Here's the drawing with two shaded views (mm, measured from the low corner). I have some questions. A direction names the side the tool comes from. Give positions to 0.01 mm unless a question says otherwise; leave off trailing zeros. Order: outer loops, then holes, each group sorted by start corner. A loop starts at its lowest first (then second) coordinate and runs counter-clockwise, first axis right, second up. Notation, with made-up numbers: (3.25, 45.25) - (53.25, 45.25) arc R17 cw to (53.25, 62.25) - close; hole circle Ø7 at (-36, 37). An arc over 180 degrees is marked (long way). Use one line per item in the form item = value. Start each with the question number.
1) Please list where these lines run through material, in increasing order: probe 1 along Y at (x, z) = (30, 11.5); probe 2 along Y at (x, z) = (30, 6.5); probe 3 along Z at (x, y) = (50, 8).
2) Which directions (+Z, -Z, +X, -X, +Y, -Y) give clear straight access to the entire face, cutting with the end or side of a thin tool? Please do the marked faces 1, 2 and 3.
3) Suppose I cut it at A-A, the plane y = 30. Write out the boundary of the cut face in (x, z).
4) Suppose I cut it at C-C, the plane z = 11.5. Write out the boundary of the cut face in (x, y), and give its area (3 significant figures).
5) Suppose I cut it at B-B, the plane z = 23.5. Write out the boundary of the cut face in (x, y).
6) We'd pull the mould along X, two halves only. Please class the marked faces 4, 5 and 6: released by +X, released by -X, zero draft, split by the parting line, or undercut.
7) For pin 1 (12 mm diameter, centred on x = 10, z = 13, fed in from +Y); pin 2 (1.5 mm diameter, centred on x = 32.5, z = 15, fed in from +Y); pin 3 (8 mm diameter, centred on x = 41, y = 37, fed in from +Z), each with a flat end and sliding along its axis, tell me the tip position at first contact or that it passes through.
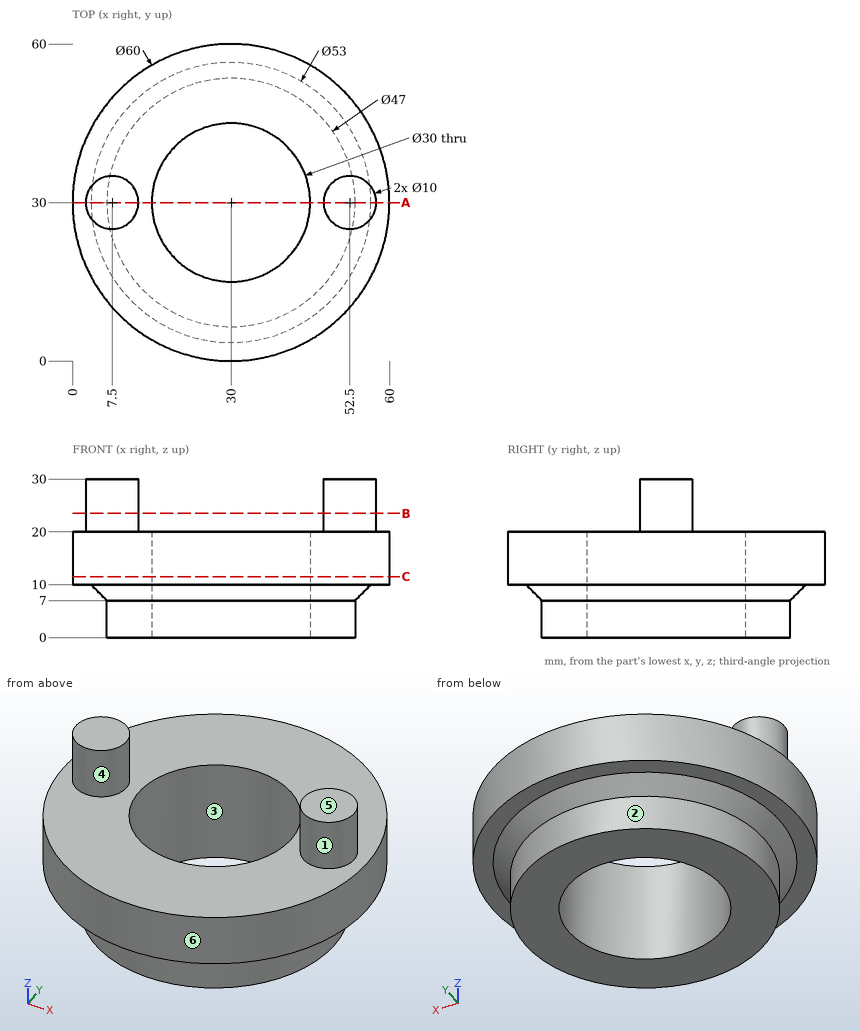
Result sheet:
q1.probe_1 = 0 to 15, 45 to 60
q1.probe_2 = 6.5 to 15, 45 to 53.5
q1.probe_3 = 10 to 20
q2.face_1 = +Z
q2.face_2 = -Z
q2.face_3 = +Z, -Z
q3.outline = (0, 10) - (3.5, 10) - (6.5, 7) - (6.5, 0) - (15, 0) - (15, 20) - (12.5, 20) - (12.5, 30) - (2.5, 30) - (2.5, 20) - (0, 20) - close; (45, 0) - (53.5, 0) - (53.5, 7) - (56.5, 10) - (60, 10) - (60, 20) - (57.5, 20) - (57.5, 30) - (47.5, 30) - (47.5, 20) - (45, 20) - close
q4.outline = circle Ø60 at (30, 30); hole circle Ø30 at (30, 30)
q4.area = 2,120 mm²
q5.outline = circle Ø10 at (7.5, 30); circle Ø10 at (52.5, 30)
q6.face_4 = undercut
q6.face_5 = zero draft
q6.face_6 = split by the parting line
q7.pin_1 = 56.53
q7.pin_2 = 59.95
q7.pin_3 = 20
